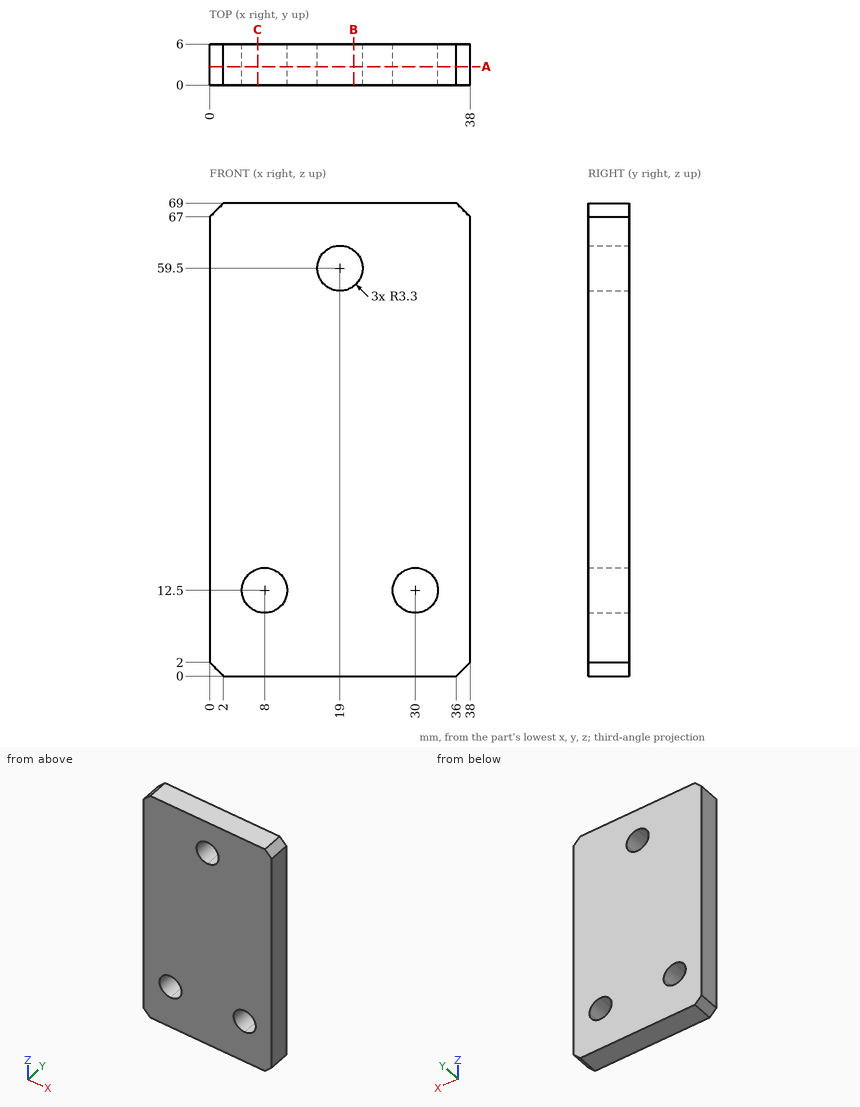
Can you work these out from the drawing? Everything is in mm from the part's minimum corner. Coordinates: 2 decimals unless noted, no trailing zeros. Write each loop counter-clockwise with the first axis right and the second up, starting at its lowest first coordinate (ties: lowest second). Pieces come first, ordered by that corner, then holes. Notation, with made-up numbers: (59, 13) -> (68, 13) arc R9 cw to (68, 17) -> close; hole circle Ø1 at (83, 22). An arc over 180 degrees is marked (long way). Write each question's results on one line, items separated by ' | '. Start each with the question number.
Q1. If I drill on probe 1 along Z at (x, y) = (10, 5.3); probe 2 along Z at (x, y) = (16.5, 2.1); probe 3 along X at (y, z) = (2.9, 58.5), over which ranges is the centre line in solid material (lowest first)?
Q2. I'm going to push a flat-ended pin straight in: pin 1 (8 mm diameter, centred on x = 10, z = 13.5, fed in from -Y). Where does the tip first touch, or does it pass through?
Q3. Imagine slicing it at C-C (x = 7). Write out the boundary of the cut face in (y, z), then the cut area to 3 significant figures.
Q4. Imagine slicing it at A-A (y = 2.7). Write out the boundary of the cut face in (x, z).
Q5. Imagine slicing it at B-B (x = 21). Write out the boundary of the cut face in (y, z).
Taken from the geometry:
1) probe 1: z = 0 to 9.88, 15.12 to 69 | probe 2: z = 0 to 57.35, 61.65 to 69 | probe 3: x = 0 to 15.86, 22.14 to 38
2) pin 1: stops at y = 0
3) outline: (0, 0) -> (6, 0) -> (6, 9.36) -> (0, 9.36) -> close; (0, 15.64) -> (6, 15.64) -> (6, 69) -> (0, 69) -> close | area: 376 mm^2
4) outline: (0, 2) -> (2, 0) -> (36, 0) -> (38, 2) -> (38, 67) -> (36, 69) -> (2, 69) -> (0, 67) -> close; hole (4.7, 12.5) arc R3.3 ccw to (8, 9.2) arc R3.3 ccw to (11.3, 12.5) arc R3.3 ccw to (8, 15.8) arc R3.3 ccw to start; hole (15.7, 59.5) arc R3.3 ccw to (19, 56.2) arc R3.3 ccw to (22.3, 59.5) arc R3.3 ccw to (19, 62.8) arc R3.3 ccw to start; hole (26.7, 12.5) arc R3.3 ccw to (30, 9.2) arc R3.3 ccw to (33.3, 12.5) arc R3.3 ccw to (30, 15.8) arc R3.3 ccw to start
5) outline: (0, 0) -> (6, 0) -> (6, 56.88) -> (0, 56.88) -> close; (0, 62.12) -> (6, 62.12) -> (6, 69) -> (0, 69) -> close
